```python
from build123d import *

# Parameters (mm, degrees)
F2_W     = 3.9979876956
F2_H     = 4
F3_DEPTH = 5
F4_W     = 8
F4_H     = 2
F4_W_2   = 2
F4_H_2   = 8
F5_DEPTH = 3.5
F6_SIZE  = 2


with BuildPart() as f1:
    # F0 (on Top) → F1 (revolve)
    with BuildSketch(Plane.XY):
        Polygon((0, 1.5), (0, 0), (6, 0), (11, 3.5), (14, 3.5), (14, 5), (10.5, 5), (10.5, 10), (9.3, 10), (9.3, 4.1409833424), (5.5271666538, 1.5), align=None)
    revolve(axis=Axis((0, 5.6900531054, 0), (0, 1, 0)))

    # F2 (on face) → F3 (cut, through all)
    with BuildSketch(Plane(origin=(0, 10, 0), x_dir=(-1, 0, 0), z_dir=(0, 1, 0))):
        with Locations((9.9453665316, 0)):
            Rectangle(F2_W, F2_H)
        Polygon((4.2401293821, 11.3441195205), (2.2411355343, 7.8817606121), (5.7052371495, 5.8817606121), (7.7042309973, 9.3441195205), align=None)
        Polygon((-7.7042309973, 9.3441195205), (-5.7052371495, 5.8817606121), (-2.2411355343, 7.8817606121), (-4.2401293821, 11.3441195205), align=None)
        with Locations((-9.9453665316, 0)):
            Rectangle(F2_W, F2_H)
        Polygon((-4.2401293821, -11.3441195205), (-2.2411355343, -7.8817606121), (-5.7052371495, -5.8817606121), (-7.7042309973, -9.3441195205), align=None)
        Polygon((7.7042309973, -9.3441195205), (5.7052371495, -5.8817606121), (2.2411355343, -7.8817606121), (4.2401293821, -11.3441195205), align=None)
    extrude(amount=-F3_DEPTH, mode=Mode.SUBTRACT)

    # F4 (on face) → F5 (join, through all)
    with BuildSketch(Plane.XZ):
        with Locations((-8, 0)):
            Rectangle(F4_W, F4_H)
        with Locations((0, -8)):
            Rectangle(F4_W_2, F4_H_2)
        with Locations((8, 0)):
            Rectangle(F4_W, F4_H)
        with Locations((0, 8)):
            Rectangle(F4_W_2, F4_H_2)
    extrude(amount=-F5_DEPTH)

    # F6
    f6_edges = [f1.edges().sort_by_distance(p)[0] for p in [
        (-12, 0, 0),
        (0, 0, -12),
        (12, 0, 0),
        (0, 0, 12),
    ]]
    chamfer(f6_edges, length=F6_SIZE)


solid = f1.part
```
Check sheet for the modelled part. Datum: model origin and axes. Units: mm. A direction names the side the tool comes from. Give positions to 0.01 mm unless a question says otherwise; leave off trailing zeros. Order: outer loops, then holes, each group sorted by start corner. A loop starts at its lowest first (then second) coordinate and runs counter-clockwise, first axis right, second up. Notation, with made-up numbers: (24.5, 52) -> (63.5, 52) arc R29 ccw to (63.5, 81) -> close; hole circle Ø2 at (-36, -29.5). An arc over 180 degrees is marked (long way). Use CSV: the item, a comma, the result in double quotes. Start each with the question number.
1) Set-up check for faces 5 (the face through (1, 1, 10)), 6 (the face through (-12, 3, 0)), 7 (the face through (6.58, 7.54, 7.4)), 8 (the face through (-4, 2, 0)), 9 (the face through (10, 8, -2)): record each of +Z, -Z, +X, -X, +Y, -Y from which the full face is reachable in a straight line by a thin tool's end or side.
2) Sectioned sample at A-A, the plane y = 9.25. Record the boundary of the cut face in (x, z).
3) Sectioned sample at B-B, the plane z = 0. Record the boundary of the cut face in (x, y), plus the area to 3 significant figures.
4) Sectioned sample at C-C, the plane x = 0. Record the boundary of the cut face in (y, z).
5) Mould release check, pull along Z, two halves, no side actions. Record for faces 1 (the face through (-3.12, 7.54, 9.4)), 2 (the face through (0, 0, -1)), 3 (the face through (5.59, 1.39, 5.7)), 4 (the face through (-6, 3, -1)): released by +Z, released by -Z, zero draft, split by the parting line, or undercut.
6) Material ranges on line 1 (Z direction, x = 0, y = 8.25); line 2 (Y direction, x = -12.25, z = -1.5); line 3 (Y direction, x = -1, z = -0.75), recorded low to high. Write a range as from..to.
7) Go/stop test with flat-tipped pins: P1, Ø3, axis at x = 9, z = -5, coming from the -Y side; P2, Ø1.6, axis at x = 6, y = 2, coming from the -Z side; P3, Ø0.6, axis at x = -7, y = 2.5, coming from the -Z side. Record where each tip stops, or that it passes through.
Recorded:
1,face 5,"+Z, +X, -Y"
1,face 6,"+Z, -Z, -X, -Y"
1,face 7,"+Z, +Y"
1,face 8,"+Y"
1,face 9,"+X, -X, +Y"
2,outline,"(-10.31, -2) arc R10.5 ccw to (-6.89, -7.93) -> (-6.27, -6.87) arc R9.3 cw to (-9.08, -2) -> close; (-10.31, 2) -> (-9.08, 2) arc R9.3 cw to (-6.27, 6.87) -> (-6.89, 7.93) arc R10.5 ccw to start; (-3.42, -9.93) arc R10.5 ccw to (3.42, -9.93) -> (2.81, -8.87) arc R9.3 cw to (-2.81, -8.87) -> close; (-3.42, 9.93) -> (-2.81, 8.87) arc R9.3 cw to (2.81, 8.87) -> (3.42, 9.93) arc R10.5 ccw to start; (6.27, -6.87) -> (6.89, -7.93) arc R10.5 ccw to (10.31, -2) -> (9.08, -2) arc R9.3 cw to start; (6.27, 6.87) arc R9.3 cw to (9.08, 2) -> (10.31, 2) arc R10.5 ccw to (6.89, 7.93) -> close"
3,outline,"(-14, 3.5) -> (-12, 3.5) -> (-12, 2) -> (-10, 0) -> (10, 0) -> (12, 2) -> (12, 3.5) -> (14, 3.5) -> (14, 5) -> (9.3, 5) -> (9.3, 4.14) -> (8.38, 3.5) -> (4, 3.5) -> (4, 1.5) -> (-4, 1.5) -> (-4, 3.5) -> (-8.38, 3.5) -> (-9.3, 4.14) -> (-9.3, 5) -> (-14, 5) -> close"
3,area,"78.7 mm2"
4,outline,"(0, -10) -> (2, -12) -> (3.5, -12) -> (3.5, -14) -> (5, -14) -> (5, -10.5) -> (10, -10.5) -> (10, -9.3) -> (4.14, -9.3) -> (3.5, -8.38) -> (3.5, -4) -> (1.5, -4) -> (1.5, 4) -> (3.5, 4) -> (3.5, 8.38) -> (4.14, 9.3) -> (10, 9.3) -> (10, 10.5) -> (5, 10.5) -> (5, 14) -> (3.5, 14) -> (3.5, 12) -> (2, 12) -> (0, 10) -> close"
5,face 1,"undercut"
5,face 2,"zero draft"
5,face 3,"released by +Z"
5,face 4,"undercut"
6,line 1,"-10.5..-9.3, 9.3..10.5"
6,line 2,"3.5..5"
6,line 3,"0..1.5"
7,P1,"y = 1.96"
7,P2,"z = -8.11"
7,P3,"z = -7.21"
